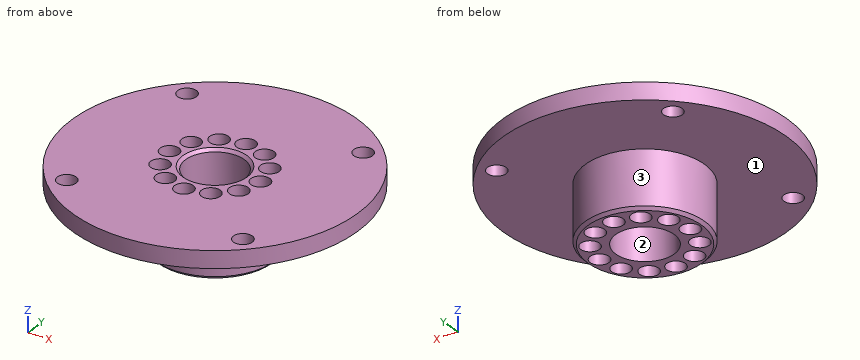
from build123d import *

# Parameters (mm, degrees)
SKETCH_R        = 10.5
PAD_DEPTH       = 10
SKETCH001_R     = 25
SKETCH001_R_2   = 1.65
PAD001_DEPTH    = 3
SKETCH002_R     = 5.15
POCKET_DEPTH    = 13.001
SKETCH003_R     = 1.65
POCKET001_DEPTH = 13.001
CHAMFER_SIZE    = 0.5
CHAMFER001_SIZE = 0.5


with BuildPart() as part:
    # Sketch → Pad (new body)
    with BuildSketch(Plane.XY):
        Circle(SKETCH_R)
    extrude(amount=PAD_DEPTH)

    # Sketch001 (on Face3 of Pad) → Pad001 (join)
    with BuildSketch(Plane.XY.offset(10)):
        Circle(SKETCH001_R)
        with Locations((-15.5, -15.5)):
            Circle(SKETCH001_R_2, mode=Mode.SUBTRACT)
        with Locations((15.5, -15.5)):
            Circle(SKETCH001_R_2, mode=Mode.SUBTRACT)
        with Locations((15.5, 15.5)):
            Circle(SKETCH001_R_2, mode=Mode.SUBTRACT)
        with Locations((-15.5, 15.5)):
            Circle(SKETCH001_R_2, mode=Mode.SUBTRACT)
    extrude(amount=PAD001_DEPTH)

    # Sketch002 (on Face3 of Pad001) → Pocket (cut, through all)
    with BuildSketch(Plane.XY.offset(13)):
        Circle(SKETCH002_R)
    extrude(amount=-POCKET_DEPTH, mode=Mode.SUBTRACT)

    # Sketch003 (on Face3 of Pocket) → Pocket001 (cut, through all)
    with BuildSketch(Plane.XY.offset(13)):
        with Locations((0, 8)):
            Circle(SKETCH003_R)
        with Locations((4, 6.928203)):
            Circle(SKETCH003_R)
        with Locations((6.928203, 4)):
            Circle(SKETCH003_R)
        with Locations((8, 0)):
            Circle(SKETCH003_R)
        with Locations((6.928203, -4)):
            Circle(SKETCH003_R)
        with Locations((4, -6.928203)):
            Circle(SKETCH003_R)
        with Locations((0, -8)):
            Circle(SKETCH003_R)
        with Locations((-4, -6.928203)):
            Circle(SKETCH003_R)
        with Locations((-6.928203, -4)):
            Circle(SKETCH003_R)
        with Locations((-8, 0)):
            Circle(SKETCH003_R)
        with Locations((-6.928203, 4)):
            Circle(SKETCH003_R)
        with Locations((-4, 6.928203)):
            Circle(SKETCH003_R)
    extrude(amount=-POCKET001_DEPTH, mode=Mode.SUBTRACT)

    # Chamfer
    chamfer_edges = [part.edges().sort_by_distance(p)[0] for p in [
        (-5.15, 0, 13),
    ]]
    chamfer(chamfer_edges, length=CHAMFER_SIZE)

    # Chamfer001
    chamfer001_edges = [part.edges().sort_by_distance(p)[0] for p in [
        (-10.5, 0, 0),
    ]]
    chamfer(chamfer001_edges, length=CHAMFER001_SIZE)


solid = part.part
For this review, take the finished solid that the model builds, in its own axes (mm). Face numbers are marked on the shaded views. Round coordinates to 2 decimals unless told otherwise and drop trailing zeros. Write each loop counter-clockwise with the first axis right and the second up, starting at its lowest first coordinate (ties: lowest second). Pieces come first, ordered by that corner, then holes. Notation, with made-up numbers: (-13, 75) -> (-6, 75) arc R8 cw to (-6, 84) -> close; hole circle Ø9 at (77.25, 2). An arc over 180 degrees is marked (long way). Put each result on its own line as item: value.
Q1. Consider section C-C on z = 6.75. Give the number of separate pieces and of enclosed holes in the cut face, and give its area (3 significant figures).
Determined:
separate pieces: 1
enclosed holes: 13
area: 160 mm^2
Q2. The part is to be moulded in two halves that separate along Y. For the marked faces 1, 2 and 3, say which applies: released by +Y, released by -Y, zero draft, split by the parting line, or undercut.
Determined:
face 1: zero draft
face 2: undercut
face 3: split by the parting line
Q3. Clearance check with flat-ended pins moving along their axes: pin 1 Ø1.5 at (x, z) = (-12, 10.5) entering from +Y; pin 2 Ø2.5 at (x, y) = (6.93, 4) entering from +Z; pin 3 Ø5.5 at (x, y) = (-15.5, -15.5) entering from -Z. State where each tip first meets the part, or that it passes through.
Determined:
pin 1: stops at y = 22.33
pin 2: passes through
pin 3: stops at z = 10
Q4. To check wall thickness, follow L1, parallel to Y at x = 0, z = 8.5; L2, parallel to Y at x = -1.5, z = 1.5; L3, parallel to X at y = 3.5, z = 3.75. State the ranges of each line that lie inside material, in increasing order. Write a range as [from, to].
Determined:
L1: y = [-10.5, -9.65], [-6.35, -5.15], [5.15, 6.35], [9.65, 10.5]
L2: y = [-10.39, -8.69], [-7.31, -4.93], [4.93, 7.31], [8.69, 10.39]
L3: x = [-9.9, -8.5], [-5.36, -3.78], [3.78, 5.36], [8.5, 9.9]
Q5. Consider section A-A on x = -15.5. State the section outline as (y, z) points, and give its area (3 significant figures).
Determined:
outline: (-19.62, 10) -> (-17.15, 10) -> (-17.15, 13) -> (-19.62, 13) -> close; (-13.85, 10) -> (13.85, 10) -> (13.85, 13) -> (-13.85, 13) -> close; (17.15, 10) -> (19.62, 10) -> (19.62, 13) -> (17.15, 13) -> close
area: 97.9 mm^2
